Verification items for the finished model (mm, model axes). A direction names the side the tool comes from. Coordinates: 2 decimals unless noted, no trailing zeros. Order: outer loops, then holes, each group sorted by start corner. A loop starts at its lowest first (then second) coordinate and runs counter-clockwise, first axis right, second up. Notation, with made-up numbers: M -33.5,65.5 L -26.5,65.5 A22 cw -26.5,75.5 Z; hole C 14.5,47.5 d4. An arc over 180 degrees is marked long. Return JSON: item names as keys, results as strings. Group by question number.
Q1. Thickness scan on probe 1 along Y at (x, z) = (7.5, -0.55); probe 2 along X at (y, z) = (-10, -0.65); probe 3 along Z at (x, y) = (1.75, -132). Record the ranges inside material, lowest first.
Q2. Access from +Z, -Z, +X, -X, +Y, -Y to the whole of each face (thin tool, end or side, straight path). Record for faces 1 (the face through (0, -108, -5)), 2 (the face through (13.8, -108, -5)).
Q3. Go/stop test with a flat-tipped pin: pin 1 Ø2.5 at (x, y) = (7.5, -40) entering from -Z. Record where the tip stops, or that it passes through.
Q4. Section check A-A, the plane x = 3.5. Enter the section's corners in (y, z), then the cut area to 3 significant figures.
Q5. Mould release check, pull along Z, two halves, no side actions. Record for faces 3 (the face through (7, -108, 0)), 4 (the face through (8, -108, -8.8)), 5 (the face through (8, 0, -9)): pulls with the +Z half, pulls with the -Z half, needs draft (parallel to the pull), parting line crosses it, or undercut.
Q6. Section check B-B, the plane y = -94. Enter the section's corners in (x, z), then the cut area to 3 significant figures.
Q7. Section check C-C, the plane z = -4. Enter the section's corners in (x, y).
Autodesk Inventor part; units mm, degrees
ref_plane "YZ Plane" through (0, 0, 0) normal (1, 0, 0) x (0, 1, 0)
ref_plane "XZ Plane" through (0, 0, 0) normal (0, 1, 0) x (-1, 0, 0)
ref_plane "XY Plane" through (0, 0, 0) normal (0, 0, 1) x (1, 0, 0)
sketch "スケッチ1" plane through (0, 0, 0) normal (0, 1, 0) x (-1, 0, 0)
  line L0 (0, 0) -> (-15, 0)
  line L1 (-15, 0) -> (-15, -10)
  line L2 (-15, -10) -> (0, -10)
  line L3 (0, -10) -> (0, 0)
  dimension "d0" = 15
  dimension "d1" = 10
extrude "押し出し1" add sketch "スケッチ1" against normal blind 220
shell "シェル1" thickness 1.2 removed faces 2 at (10, 0, -3.3333) at (10, -220, -3.3333)
sketch "スケッチ2" plane through (0, 0, 0) normal (0, 0, 1) x (1, 0, 0)
  line L0 (0, 0) -> (15, 0)
  line L1 (15, 0) -> (15, -220)
  line L2 (15, -220) -> (0, -220)
  point P0 (7.5, -10)
  point P1 (7.5, 0)
  point P2 (7.5, -40)
  point P3 (7.5, -210)
  point P4 (7.5, -210)
  point P5 (7.5, -180)
  dimension "d5" = 10
  dimension "d6" = 7.5
  dimension "d7" = 7.5
  dimension "d8" = 30
  dimension "d9" = 10
  dimension "d10" = 7.5
  dimension "d11" = 30
  dimension "d12" = 7.5
hole "穴1" at (7.5, -10, 0) at (7.5, -40, 0) at (7.5, -210, 0) at (7.5, -180, 0) direction (0, 0, -1) diameter 3.2 end through all
properties part number "left_ASP" material "アルミニウム 6061"
Numbers:
{
 "1": {"probe 1": "y = -220 to -211.6, -208.4 to -181.6, -178.4 to -41.6, -38.4 to -11.6, -8.4 to 0", "probe 2": "x = 0 to 5.9, 9.1 to 15", "probe 3": "z = -10 to -8.8, -1.2 to 0"},
 "2": {"face 1": "+Z, -Z, -X, +Y, -Y", "face 2": "+Y, -Y"},
 "3": {"pin 1": "passes through"},
 "4": {"outline": "M -220,-10 L 0,-10 L 0,-8.8 L -220,-8.8 Z; M -220,-1.2 L 0,-1.2 L 0,0 L -220,0 Z", "area": "528 mm2"},
 "5": {"face 3": "pulls with the +Z half", "face 4": "undercut", "face 5": "needs draft"},
 "6": {"outline": "M 0,-10 L 15,-10 L 15,0 L 0,0 Z; hole M 1.2,-8.8 L 13.8,-8.8 L 13.8,-1.2 L 1.2,-1.2 Z", "area": "54.2 mm2"},
 "7": {"outline": "M 0,-220 L 1.2,-220 L 1.2,0 L 0,0 Z; M 13.8,-220 L 15,-220 L 15,0 L 13.8,0 Z"}
}
